Model file for the job. Use its own axes, mm. Face numbers are marked on the shaded views. A direction names the side the tool comes from. Round coordinates to 2 decimals unless told otherwise and drop trailing zeros. Order: outer loops, then holes, each group sorted by start corner. A loop starts at its lowest first (then second) coordinate and runs counter-clockwise, first axis right, second up. Notation, with made-up numbers: (-32.75, 73.5) -> (-19.75, 73.5) arc R32 ccw to (-19.75, 107.5) -> close; hole circle Ø11 at (-6, 69.5). An arc over 180 degrees is marked (long way). Put each result on its own line as item: value. Start each with the question number.
Q1. Flat gauge pins, fed straight in: P1, Ø12, axis at x = 15, z = -27, coming from the -Y side; P2, Ø0.9, axis at x = 21, y = 48, coming from the -Z side; P3, Ø0.5, axis at x = 21, z = -23.5, coming from the +Y side; P4, Ø5, axis at x = 24, z = -6, coming from the +Y side. Where does each tip first touch, or does it go through?
Q2. Probe L1, parallel to X at y = 9, z = -7; L2, parallel to Z at x = 37, y = 25; L3, parallel to Z at x = 36, y = 8.5. List the from-to ranges inside material, lowest first.
Q3. Cut at D-D, the plane y = 7.5. List the corners of the cut face in (x, z) (3 decimals).
Q4. Cut at A-A, the plane z = -5. List the corners of the cut face in (x, y).
Q5. Cut at B-B, the plane x = 21.15. List the corners of the cut face in (y, z).
Q6. Cut at C-C, the plane z = -22. List the corners of the cut face in (x, y).
Q7. 3-axis set-ups, long thin cutter, end or side, ignore diameter. For the marked faces 1 and 2: which of +Z, -Z, +X, -X, +Y, -Y reach the whole face in a straight line?
from build123d import *

# Parameters (mm, degrees)
SKETCH2_W           = 42.3
SKETCH2_H           = 42.3
SKETCH2_R           = 1.5
BOSS_EXTRUDE1_DEPTH = 34
SKETCH3_R           = 11
BOSS_EXTRUDE2_DEPTH = 2.03
SKETCH4_R           = 2.5
BOSS_EXTRUDE3_DEPTH = 21.85
CUT_EXTRUDE1_START  = -14.86
CUT_EXTRUDE1_DEPTH  = 14.86
FILLET1_R           = 3
FILLET2_R           = 0.5


with BuildPart() as part:
    # Sketch2 → Boss-Extrude1 (new body)
    with BuildSketch(Plane(origin=(0, 0, 0), x_dir=(1, 0, 0), z_dir=(0, 1, 0))):
        with Locations((21.15, 21.15)):
            Rectangle(SKETCH2_W, SKETCH2_H)
        with Locations(Location((5.655, 36.645, 0), (0, 0, 270))):
            Circle(SKETCH2_R, mode=Mode.SUBTRACT)
        with Locations(Location((36.645, 36.645, 0), (0, 0, 270))):
            Circle(SKETCH2_R, mode=Mode.SUBTRACT)
        with Locations(Location((36.645, 5.655, 0), (0, 0, 270))):
            Circle(SKETCH2_R, mode=Mode.SUBTRACT)
        with Locations(Location((5.655, 5.655, 0), (0, 0, 270))):
            Circle(SKETCH2_R, mode=Mode.SUBTRACT)
    extrude(amount=BOSS_EXTRUDE1_DEPTH)

    # Sketch3 → Boss-Extrude2 (add)
    with BuildSketch(Plane(origin=(0, 34, 0), x_dir=(1, 0, 0), z_dir=(0, 1, 0))):
        with Locations(Location((21.15, 21.15, 0), (0, 0, 270))):
            Circle(SKETCH3_R)
    extrude(amount=BOSS_EXTRUDE2_DEPTH)

    # Sketch4 → Boss-Extrude3 (add)
    with BuildSketch(Plane(origin=(0, 36.03, 0), x_dir=(1, 0, 0), z_dir=(0, 1, 0))):
        with Locations(Location((21.15, 21.15, 0), (0, 0, 270))):
            Circle(SKETCH4_R)
    extrude(amount=BOSS_EXTRUDE3_DEPTH)

    # Sketch5 → Cut-Extrude1 (cut)
    with BuildSketch(Plane(origin=(0, 57.88, 0), x_dir=(1, 0, 0), z_dir=(0, 1, 0)).offset(CUT_EXTRUDE1_START)):
        with BuildLine():
            Line((19.677043789, 23.17), (22.622956211, 23.17))
            ThreePointArc((22.622956211, 23.17), (21.15, 23.65), (19.677043789, 23.17))
        make_face()
    extrude(amount=CUT_EXTRUDE1_DEPTH, mode=Mode.SUBTRACT)

    # Fillet1
    fillet1_edges = [part.edges().sort_by_distance(p)[0] for p in [
        (0, 17, -42.3),
        (42.3, 17, -42.3),
        (42.3, 17, 0),
        (0, 17, 0),
    ]]
    fillet(fillet1_edges, radius=FILLET1_R)

    # Fillet2
    fillet2_edges = [part.edges().sort_by_distance(p)[0] for p in [
        (0, 0, -21.15),
        (0, 34, -21.15),
        (21.15, 0, -42.3),
        (42.3, 0, -21.15),
        (21.15, 0, 0),
        (0.878679656, 0, -0.878679656),
        (41.421320344, 0, -0.878679656),
        (41.421320344, 0, -41.421320344),
        (0.878679656, 0, -41.421320344),
        (21.15, 34, -42.3),
        (21.15, 34, 0),
        (42.3, 34, -21.15),
        (0.878679656, 34, -0.878679656),
        (41.421320344, 34, -0.878679656),
        (41.421320344, 34, -41.421320344),
        (0.878679656, 34, -41.421320344),
    ]]
    fillet(fillet2_edges, radius=FILLET2_R)


solid = part.part
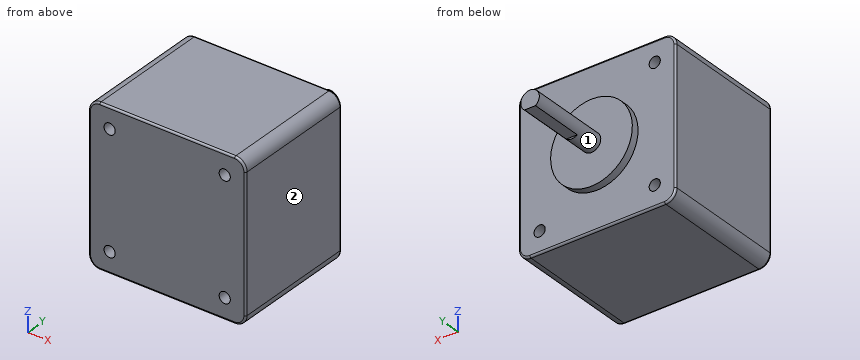
Ans:
1. P1: stops at y = 0
1. P2: stops at z = -23.17
1. P3: stops at y = 43.02
1. P4: stops at y = 34
2. L1: x = 0 to 4.99, 6.32 to 35.98, 37.31 to 42.3
2. L2: z = -42.3 to -38.1, -35.19 to -7.11, -4.2 to 0
2. L3: z = -42.3 to -38, -35.29 to -7.01, -4.3 to 0
3. outline: (0, -39.3) arc R3 ccw to (3, -42.3) -> (39.3, -42.3) arc R3 ccw to (42.3, -39.3) -> (42.3, -3) arc R3 ccw to (39.3, 0) -> (3, 0) arc R3 ccw to (0, -3) -> close; hole circle Ø3 at (5.655, -36.645); hole circle Ø3 at (5.655, -5.655); hole circle Ø3 at (36.645, -36.645); hole circle Ø3 at (36.645, -5.655)
4. outline: (0, 0.5) arc R0.5 ccw to (0.5, 0) -> (4.31, 0) -> (4.31, 34) -> (0.5, 34) arc R0.5 ccw to (0, 33.5) -> close; (7, 0) -> (35.3, 0) -> (35.3, 34) -> (7, 34) -> close; (37.99, 0) -> (41.8, 0) arc R0.5 ccw to (42.3, 0.5) -> (42.3, 33.5) arc R0.5 ccw to (41.8, 34) -> (37.99, 34) -> close
5. outline: (0, -41.8) arc R0.5 ccw to (0.5, -42.3) -> (33.5, -42.3) arc R0.5 ccw to (34, -41.8) -> (34, -32.15) -> (36.03, -32.15) -> (36.03, -23.65) -> (43.02, -23.65) -> (43.02, -23.17) -> (57.88, -23.17) -> (57.88, -18.65) -> (36.03, -18.65) -> (36.03, -10.15) -> (34, -10.15) -> (34, -0.5) arc R0.5 ccw to (33.5, 0) -> (0.5, 0) arc R0.5 ccw to (0, -0.5) -> close
6. outline: (0, 0.5) arc R0.5 ccw to (0.5, 0) -> (41.8, 0) arc R0.5 ccw to (42.3, 0.5) -> (42.3, 33.5) arc R0.5 ccw to (41.8, 34) -> (32.12, 34) -> (32.12, 36.03) -> (23.5, 36.03) -> (23.5, 57.88) -> (18.8, 57.88) -> (18.8, 36.03) -> (10.18, 36.03) -> (10.18, 34) -> (0.5, 34) arc R0.5 ccw to (0, 33.5) -> close
7. face 1: +Y
7. face 2: +Z, -Z, +X, +Y, -Y
